```python
from build123d import *

# Parameters (mm, degrees)
SKETCH1_R            = 15
SKETCH1_R_2          = 10
BOSS_EXTRUDE1_DEPTH  = 80
BOSS_EXTRUDE2_DEPTH  = 5
BOSS_EXTRUDE3_DEPTH  = 15
BOSS_EXTRUDE21_DEPTH = 2.5
CUT_EXTRUDE1_DEPTH   = 15
CUT_EXTRUDE2_DEPTH   = 80


with BuildPart() as part:
    # Sketch1 → Boss-Extrude1 (new body)
    with BuildSketch(Plane.XY):
        Circle(SKETCH1_R)
        Circle(SKETCH1_R_2, mode=Mode.SUBTRACT)
    extrude(amount=BOSS_EXTRUDE1_DEPTH)

    # Sketch1_3 → Boss-Extrude2 (add)
    with BuildSketch(Plane.XY):
        with BuildLine():
            Line((-15, 0), (-15, -7.5))
            ThreePointArc((-15, -7.5), (0, -22.5), (15, -7.5))
            Line((15, -7.5), (15, 0))
            ThreePointArc((15, 0), (0, -15), (-15, 0))
        make_face()
    extrude(amount=BOSS_EXTRUDE2_DEPTH)

    # Sketch2 → Boss-Extrude3 (add, symmetric)
    with BuildSketch(Plane(origin=(0, 0, 0), x_dir=(0, 0, -1), z_dir=(1, 0, 0))):
        with BuildLine():
            Line((-80, 25), (-80, 0))
            Line((-80, 0), (-60, 0))
            Line((-60, 0), (-60, 10.857864376))
            ThreePointArc((-60, 10.857864376), (-51.277883135, 18.941657921), (-51.180759566, 30.83340328))
            Line((-51.180759566, 30.83340328), (-5, 15))
            Line((-5, 15), (-5, 0))
            Line((-5, 0), (0, 0))
            Line((0, 0), (0, 15))
            Line((0, 15), (0, 20))
            Line((0, 20), (-60.439243158, 39.289838943))
            ThreePointArc((-60.439243158, 39.289838943), (-73.848407975, 37.112211867), (-80, 25))
        make_face()
        with BuildLine():
            Line((-67.5, 15.317541634), (-67.5, 7.5))
            Line((-67.5, 7.5), (-62.5, 7.5))
            Line((-62.5, 7.5), (-62.5, 15.317541634))
            ThreePointArc((-62.5, 15.317541634), (-65, 35), (-67.5, 15.317541634))
        make_face(mode=Mode.SUBTRACT)
    extrude(amount=BOSS_EXTRUDE3_DEPTH, both=True)

    # Sketch2_8 → Boss-Extrude21 (add, symmetric)
    with BuildSketch(Plane(origin=(0, 0, 0), x_dir=(0, 0, -1), z_dir=(1, 0, 0))):
        with BuildLine():
            Line((-60, 10.857864376), (-60, 10))
            Line((-60, 10), (-5, 10))
            Line((-5, 10), (-5, 15))
            Line((-5, 15), (-51.180759566, 30.83340328))
            ThreePointArc((-51.180759566, 30.83340328), (-51.277883135, 18.941657921), (-60, 10.857864376))
        make_face()
    extrude(amount=BOSS_EXTRUDE21_DEPTH, both=True)

    # Sketch2_9 → Cut-Extrude1 (cut, symmetric)
    with BuildSketch(Plane(origin=(0, 0, 0), x_dir=(0, 0, -1), z_dir=(1, 0, 0))):
        with BuildLine():
            Line((-62.5, 7.5), (-62.5, 15.317541634))
            ThreePointArc((-62.5, 15.317541634), (-65, 35), (-67.5, 15.317541634))
            Line((-67.5, 15.317541634), (-67.5, 7.5))
            Line((-67.5, 7.5), (-62.5, 7.5))
        make_face()
    extrude(amount=CUT_EXTRUDE1_DEPTH, both=True, mode=Mode.SUBTRACT)

    # Sketch1_4 → Cut-Extrude2 (cut)
    with BuildSketch(Plane.XY):
        with BuildLine():
            Line((0, 0), (10, 0))
            ThreePointArc((10, 0), (0, 10), (-10, 0))
            Line((-10, 0), (0, 0))
        make_face()
    extrude(amount=CUT_EXTRUDE2_DEPTH, mode=Mode.SUBTRACT)


solid = part.part
```
Check sheet for the modelled part. Datum: model origin and axes. Units: mm. A direction names the side the tool comes from. Give positions to 0.01 mm unless a question says otherwise; leave off trailing zeros. Order: outer loops, then holes, each group sorted by start corner. A loop starts at its lowest first (then second) coordinate and runs counter-clockwise, first axis right, second up. Notation, with made-up numbers: (-40, -37.5) -> (9, -37.5) arc R12 cw to (9, -28.5) -> close; hole circle Ø11 at (52, -5). An arc over 180 degrees is marked (long way). Return JSON: item names as keys, results as strings.
1. Set-up check for faces 1 (the flat face through (2.5, 19, 35)), 2 (the flat face through (-2.5, 19, 35)), 3 (the cylindrical face through (-2.17, -9.76, 39.44)), 4 (the flat face through (0, 11, 67.5)): record each of +Z, -Z, +X, -X, +Y, -Y from which the full face is reachable in a straight line by a thin tool's end or side.
From the geometry:
{"face 1": "+X", "face 2": "-X", "face 3": "+Z, -Z", "face 4": "+X, -X"}
2. Cross-section at C-C, the plane x = 4. Record the cut outline in (y, z).
From the geometry:
{"outline": "(-21.96, 0) -> (-9.17, 0) -> (-9.17, 80) -> (-14.46, 80) -> (-14.46, 5) -> (-21.96, 5) -> close; (9.17, 0) -> (20, 0) -> (39.29, 60.44) arc R15 ccw to (25, 80) -> (9.17, 80) -> (9.17, 67.5) -> (15.32, 67.5) arc R10 cw (long way) to (15.32, 62.5) -> (9.17, 62.5) -> close; hole (14.46, 5) -> (15, 5) -> (30.83, 51.18) arc R15 cw to (14.46, 54.33) -> close"}
3. Cross-section at A-A, the plane z = 65. Record the cut outline in (x, y).
From the geometry:
{"outline": "(-15, 0) arc R15 ccw to (15, 0) -> (15, 7.5) -> (6.61, 7.5) arc R10 cw (long way) to (-6.61, 7.5) -> (-15, 7.5) -> close; (-15, 35) -> (15, 35) -> (15, 40) -> (-15, 40) -> close"}
4. Go/stop test with flat-tipped pins: P1, Ø2, axis at y = 3, z = 31, coming from the +X side; P2, Ø2, axis at x = 7, z = 35, coming from the -Y side; P3, Ø2.5, axis at x = -12, y = 7, coming from the -Z side; P4, Ø1.5, axis at y = 11, z = 35.5, coming from the -X side. Record where each tip stops, or that it passes through.
From the geometry:
{"P1": "x = 14.87", "P2": "y = -13.75", "P3": "z = 0", "P4": "x = -10.95"}
5. Cross-section at B-B, the plane x = 0. Record the cut outline in (y, z).
From the geometry:
{"outline": "(-22.5, 0) -> (-10, 0) -> (-10, 80) -> (-15, 80) -> (-15, 5) -> (-22.5, 5) -> close; (10, 0) -> (20, 0) -> (39.29, 60.44) arc R15 ccw to (25, 80) -> (10, 80) -> (10, 67.5) -> (15.32, 67.5) arc R10 cw (long way) to (15.32, 62.5) -> (10, 62.5) -> close"}
6. Material ranges on probe 1 along Y at (x, z) = (8.75, 65); probe 2 along X at (y, z) = (0, 39.5); probe 3 along Y at (x, z) = (12, 58.5), recorded low to high. Write a range as [from, to].
From the geometry:
{"probe 1": "[-12.18, -4.84], [4.84, 7.5], [35, 40]", "probe 2": "[-15, -10], [10, 15]", "probe 3": "[-9, 9], [11.48, 17.4], [32.6, 38.67]"}
7. Mould release check, pull along Y, two halves, no side actions. Record for faces 5 (the flat face through (-11, 7.5, 65)), 6 (the cylindrical face through (-0.33, -22.496, 2.465)), 7 (the flat face through (0.21, 29.51, 29.8)): +Y half, -Y half, draft (parallel to the pull), parting line (faces both ways), or undercut.
From the geometry:
{"face 5": "undercut", "face 6": "-Y half", "face 7": "+Y half"}
8. Cross-section at D-D, the plane z = 28.5. Record the cut outline in (x, y).
From the geometry:
{"outline": "(-15, 23.06) -> (-2.5, 23.06) -> (-2.5, 14.79) arc R15 ccw (long way) to (2.5, 14.79) -> (2.5, 23.06) -> (15, 23.06) -> (15, 29.1) -> (-15, 29.1) -> close; hole circle Ø20 at (0, 0)"}
